Build history of the part. All positions in model axes, mm. A direction names the side the tool comes from. Coordinates: 2 decimals unless noted, no trailing zeros. Write each loop counter-clockwise with the first axis right and the second up, starting at its lowest first coordinate (ties: lowest second). Pieces come first, ordered by that corner, then holes.
from build123d import *

# Parameters (mm, degrees)
BASPROSKE_W         = 10
BASPROSKE_H         = 13.5
TOOTHCUT_DEPTH      = 22.552262062
TEETHCUTS_COUNT     = 16
TEETHCUTS_ANGLE     = 337.5
BORSKE_R            = 3
BORE_DEPTH          = 50.0000508
KEYSKE_W            = 2
KEYSKE_H            = 4
KEYWAY_DEPTH        = 50.0000508
SKETCH1_R           = 5.698738584
BOSS_EXTRUDE1_DEPTH = 10


with BuildPart() as part:
    # BasProSke → Base-Revolve (revolve)
    with BuildSketch(Plane(origin=(0, 0, 0), x_dir=(1, 0, 0), z_dir=(0, 1, 0)), mode=Mode.PRIVATE) as base_revolve_sk:
        with Locations((5, 6.75)):
            Rectangle(BASPROSKE_W, BASPROSKE_H)
    revolve(base_revolve_sk.sketch.rotate(Axis((-10, 0, 0), (1, 0, 0)), 180), axis=Axis((-10, 0, 0), (1, 0, 0)))

    # TooCutSke → ToothCut (cut, through all)
    with BuildSketch(Plane(origin=(0, 0, 0), x_dir=(0, 0, -1), z_dir=(1, 0, 0))):
        with BuildLine():
            ThreePointArc((0.91215808, 10.08282419), (0, 10.124), (-0.91215808, 10.08282419))
            ThreePointArc((-0.91215808, 10.08282419), (-1.23025345, 11.835184302), (-2.165362868, 13.35094187))
            ThreePointArc((-2.165362868, 13.35094187), (0, 13.5254), (2.165362868, 13.35094187))
            ThreePointArc((2.165362868, 13.35094187), (1.23025345, 11.835184302), (0.91215808, 10.08282419))
        make_face()
    toothcut = extrude(amount=TOOTHCUT_DEPTH, mode=Mode.SUBTRACT)

    # TeethCuts: ToothCut ×16 about axis
    teethcuts_axis = Axis((-10, 0, 0), (1, 0, 0))
    for i in range(1, TEETHCUTS_COUNT):
        add(toothcut.rotate(teethcuts_axis, i * TEETHCUTS_ANGLE / (TEETHCUTS_COUNT - 1)), mode=Mode.SUBTRACT)

    # BorSke → Bore (cut, symmetric)
    with BuildSketch(Plane(origin=(0, 0, 0), x_dir=(0, 0, -1), z_dir=(1, 0, 0))):
        with Locations(Location((0, 0, 0), (0, 0, 180))):
            Circle(BORSKE_R)
    extrude(amount=BORE_DEPTH, both=True, mode=Mode.SUBTRACT)

    # KeySke → Keyway (cut, symmetric)
    with BuildSketch(Plane(origin=(0, 0, 0), x_dir=(0, 0, -1), z_dir=(1, 0, 0))):
        with Locations((0, 2)):
            Rectangle(KEYSKE_W, KEYSKE_H)
    extrude(amount=KEYWAY_DEPTH, both=True, mode=Mode.SUBTRACT)

    # Sketch1 → Boss-Extrude1 (add, through all)
    with BuildSketch(Plane(origin=(10, 0, 0), x_dir=(0, 0, -1), z_dir=(1, 0, 0))):
        Circle(SKETCH1_R)
        with BuildLine():
            Line((-1, 4), (-1, 1.2489996))
            ThreePointArc((-1, 1.2489996), (0, -1.6), (1, 1.2489996))
            Line((1, 1.2489996), (1, 4))
            Line((1, 4), (-1, 4))
        make_face(mode=Mode.SUBTRACT)
    extrude(amount=-BOSS_EXTRUDE1_DEPTH)


solid = part.part
(1) Flat gauge pins, fed straight in: P1, Ø1, axis at x = 1.5, y = 8.5, coming from the -Z side; P2, Ø1.5, axis at x = 6.5, y = 5, coming from the -Z side; P3, Ø0.8, axis at x = 6, y = 3, coming from the +Z side. Where does each tip first touch, or does it go through?
(2) 3-axis set-ups, long thin cutter, end or side, ignore diameter. For faces 1 (the cylindrical face through (4.93, -7.15, 7.17)), 2 (the cylindrical face through (4.9, -5.7, -10.5)), 3 (the cylindrical face through (4.9, 5.7, 10.5)): which of +Z, -Z, +X, -X, +Y, -Y reach the whole face in a straight line?
(3) Slice it at A-A, the plane z = 0. List the corners of the cut face in (x, y), and give its area (3 significant figures).
(4) Slice it at B-B, the plane y = 0. List the corners of the cut face in (x, z), and give its area (3 significant figures).
(5) Two-plate mould, pull along Y, no slides. Class faces 4 (the cylindrical face through (5.07, 11.23, 7.49)), 5 (the cylindrical face through (5.07, -11.22, 7.51)), 6 (the cylindrical face through (4.93, 7.17, 7.15)): pulls with the +Y half, pulls with the -Y half, needs draft (parallel to the pull), parting line crosses it, or undercut.
(6) Probe L1, parallel to Y at x = 5.5, z = 0; L2, parallel to Z at x = 6.25, y = 0; L3, parallel to Y at x = 9.25, z = -0.75. List the from-to ranges inside material, lowest first.
(7) Slice it at C-C, the plane z = -6. List the corners of the cut face in (x, y), and give its area (3 significant figures).
Results:
1. P1: stops at z = -7.38
1. P2: stops at z = -10.55
1. P3: stops at z = 13.25
2. face 1: +X, -X
2. face 2: -Z, +X, -X
2. face 3: +Z, +X, -X
3. outline: (0, -10.12) - (10, -10.12) - (10, -1.6) - (0, -1.6) - close; (0, 4) - (10, 4) - (10, 10.12) - (0, 10.12) - close
3. area: 146 mm2
4. outline: (0, -10.12) - (10, -10.12) - (10, -1.6) - (0, -1.6) - close; (0, 1.6) - (10, 1.6) - (10, 10.12) - (0, 10.12) - close
4. area: 170 mm2
5. face 4: pulls with the +Y half
5. face 5: pulls with the -Y half
5. face 6: undercut
6. L1: y = -10.12 to -1.6, 4 to 10.12
6. L2: z = -10.12 to -1.6, 1.6 to 10.12
6. L3: y = -10.1 to -1.41, 4 to 10.1
7. outline: (0, -10.78) - (10, -10.78) - (10, 10.78) - (0, 10.78) - close
7. area: 216 mm2
